The model under review builds one solid part; all positions refer to its coordinate system, in mm. Face numbers are marked on the shaded views. A direction names the side the tool comes from. Round coordinates to 2 decimals unless told otherwise and drop trailing zeros. Write each loop counter-clockwise with the first axis right and the second up, starting at its lowest first coordinate (ties: lowest second). Pieces come first, ordered by that corner, then holes. Notation, with made-up numbers: (24, 63.5) - (76, 63.5) arc R28 cw to (76, 96.5) - close; hole circle Ø4 at (38.5, 55.5). An arc over 180 degrees is marked (long way). Return JSON: item names as keys, results as strings.
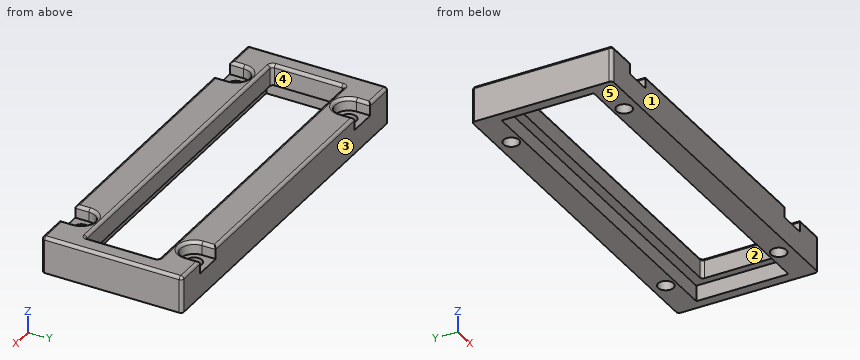
from build123d import *

# Parameters (mm, degrees)
SKETCH1_W                                      = 63.5
SKETCH1_H                                      = 24.384
BOSS_EXTRUDE1_DEPTH                            = 6.35
CBORE_FOR_2_SOCKET_HEAD_CAP_SCREW1_D           = 2.7051
CBORE_FOR_2_SOCKET_HEAD_CAP_SCREW1_CBORE_D     = 4.7625
CBORE_FOR_2_SOCKET_HEAD_CAP_SCREW1_CBORE_DEPTH = 2.1844
SKETCH4_W                                      = 57.404
SKETCH4_H                                      = 12.7
CUT_EXTRUDE1_DEPTH                             = 7.35
SKETCH5_W                                      = 4.7625
SKETCH5_H                                      = 2.3876
CUT_EXTRUDE2_DEPTH                             = 2.1844
SKETCH7_W                                      = 57.404
SKETCH7_H                                      = 12.7
CUT_EXTRUDE3_DEPTH                             = 2.7432
FILLET1_R                                      = 0.508
SKETCH11_W                                     = 60
SKETCH11_H                                     = 16
CUT_EXTRUDE6_DEPTH                             = 3.7432
BOSS_EXTRUDE2_REACH                            = 8.35


with BuildPart() as part:
    # Sketch1 → Boss-Extrude1 (new body)
    with BuildSketch(Plane.XY):
        with Locations((137.237805359, -177.626597764)):
            Rectangle(SKETCH1_W, SKETCH1_H)
    extrude(amount=BOSS_EXTRUDE1_DEPTH)

    # CBORE for #2 Socket Head Cap Screw1 (through all)
    with Locations(Plane.XY.offset(6.35)):
        with Locations((161.050305359, -187.430997764), (113.425305359, -187.430997764), (161.050305359, -167.822197764), (113.425305359, -167.822197764)):
            CounterBoreHole(CBORE_FOR_2_SOCKET_HEAD_CAP_SCREW1_D / 2, CBORE_FOR_2_SOCKET_HEAD_CAP_SCREW1_CBORE_D / 2, CBORE_FOR_2_SOCKET_HEAD_CAP_SCREW1_CBORE_DEPTH)

    # Sketch4 → Cut-Extrude1 (cut, through all)
    with BuildSketch(Plane.XY.offset(6.35)):
        with Locations((137.237805359, -177.626597764)):
            Rectangle(SKETCH4_W, SKETCH4_H)
    extrude(amount=-CUT_EXTRUDE1_DEPTH, mode=Mode.SUBTRACT)

    # Sketch5 → Cut-Extrude2 (cut)
    with BuildSketch(Plane.XY.offset(6.35)):
        with Locations((113.425305359, -166.628397764)):
            Rectangle(SKETCH5_W, SKETCH5_H)
        with Locations((161.050305359, -166.628397764)):
            Rectangle(SKETCH5_W, SKETCH5_H)
        with Locations((113.425305359, -188.624797764)):
            Rectangle(SKETCH5_W, SKETCH5_H)
        with Locations((161.050305359, -188.624797764)):
            Rectangle(SKETCH5_W, SKETCH5_H)
    extrude(amount=-CUT_EXTRUDE2_DEPTH, mode=Mode.SUBTRACT)

    # Sketch7 → Cut-Extrude3 (cut)
    with BuildSketch(Plane(origin=(0, 0, 0), x_dir=(-1, 0, 0), z_dir=(0, 0, -1))):
        with BuildLine():
            Line((-163.431555359, -167.822197764), (-163.431555359, -166.704597764))
            Line((-163.431555359, -166.704597764), (-167.717805359, -166.704597764))
            Line((-167.717805359, -166.704597764), (-167.717805359, -188.548597764))
            Line((-167.717805359, -188.548597764), (-163.431555359, -188.548597764))
            Line((-163.431555359, -188.548597764), (-163.431555359, -187.430997764))
            ThreePointArc((-163.431555359, -187.430997764), (-161.050305359, -185.049747764), (-158.669055359, -187.430997764))
            Line((-158.669055359, -187.430997764), (-158.669055359, -188.548597764))
            Line((-158.669055359, -188.548597764), (-115.806555359, -188.548597764))
            Line((-115.806555359, -188.548597764), (-115.806555359, -187.430997764))
            ThreePointArc((-115.806555359, -187.430997764), (-113.425305359, -185.049747764), (-111.044055359, -187.430997764))
            Line((-111.044055359, -187.430997764), (-111.044055359, -188.548597764))
            Line((-111.044055359, -188.548597764), (-106.757805359, -188.548597764))
            Line((-106.757805359, -188.548597764), (-106.757805359, -166.704597764))
            Line((-106.757805359, -166.704597764), (-111.044055359, -166.704597764))
            Line((-111.044055359, -166.704597764), (-111.044055359, -167.822197764))
            ThreePointArc((-111.044055359, -167.822197764), (-113.425305359, -170.203447764), (-115.806555359, -167.822197764))
            Line((-115.806555359, -167.822197764), (-115.806555359, -166.704597764))
            Line((-115.806555359, -166.704597764), (-158.669055359, -166.704597764))
            Line((-158.669055359, -166.704597764), (-158.669055359, -167.822197764))
            ThreePointArc((-158.669055359, -167.822197764), (-161.050305359, -170.203447764), (-163.431555359, -167.822197764))
        make_face()
        with Locations((-137.237805359, -177.626597764)):
            Rectangle(SKETCH7_W, SKETCH7_H, mode=Mode.SUBTRACT)
    extrude(amount=-CUT_EXTRUDE3_DEPTH, mode=Mode.SUBTRACT)

    # Fillet1
    fillet1_edges = [part.edges().sort_by_distance(p)[0] for p in [
        (105.487805359, -177.626597764, 6.35),
        (166.209680359, -189.818597764, 6.35),
        (158.669055359, -188.624797764, 6.35),
        (163.431555359, -188.624797764, 6.35),
        (108.265930359, -189.818597764, 6.35),
        (108.535805359, -171.276597764, 4.5466),
        (165.939805359, -171.276597764, 4.5466),
        (108.535805359, -183.976597764, 4.5466),
        (165.939805359, -183.976597764, 4.5466),
        (106.757805359, -166.704597764, 1.3716),
        (111.044055359, -166.704597764, 1.3716),
        (115.806555359, -166.704597764, 1.3716),
        (113.425305359, -185.049747764, 6.35),
        (161.050305359, -185.049747764, 6.35),
        (168.987805359, -177.626597764, 6.35),
        (165.939805359, -177.626597764, 6.35),
        (137.237805359, -171.276597764, 6.35),
        (108.535805359, -177.626597764, 6.35),
        (137.237805359, -183.976597764, 6.35),
        (113.425305359, -170.203447764, 6.35),
        (108.265930359, -165.434597764, 6.35),
        (115.806555359, -166.628397764, 6.35),
        (111.044055359, -166.628397764, 6.35),
        (166.209680359, -165.434597764, 6.35),
        (168.987805359, -189.818597764, 3.175),
        (105.487805359, -189.818597764, 3.175),
        (161.050305359, -170.203447764, 6.35),
        (105.487805359, -165.434597764, 3.175),
        (168.987805359, -165.434597764, 3.175),
        (137.237805359, -165.434597764, 6.35),
        (163.431555359, -166.628397764, 6.35),
        (158.669055359, -166.628397764, 6.35),
        (137.237805359, -189.818597764, 6.35),
        (115.806555359, -188.624797764, 6.35),
        (111.044055359, -188.624797764, 6.35),
    ]]
    fillet(fillet1_edges, radius=FILLET1_R)

    # Sketch11 → Cut-Extrude6 (cut, through all)
    with BuildSketch(Plane(origin=(0, 0, 2.7432), x_dir=(-1, 0, 0), z_dir=(0, 0, -1))):
        with Locations((-137.237805359, -177.626597764)):
            Rectangle(SKETCH11_W, SKETCH11_H)
    extrude(amount=CUT_EXTRUDE6_DEPTH, mode=Mode.SUBTRACT)

    # Sketch10 → Boss-Extrude2 (add, up to next)
    with BuildSketch(Plane(origin=(0, 0, 0), x_dir=(-1, 0, 0), z_dir=(0, 0, -1)), mode=Mode.PRIVATE) as boss_extrude2_sk1:
        with BuildLine():
            ThreePointArc((-158.669055359, -167.822197764), (-158.885762757, -168.814723274), (-159.496441722, -169.626597764))
            Line((-159.496441722, -169.626597764), (-114.979168996, -169.626597764))
            ThreePointArc((-114.979168996, -169.626597764), (-115.58984796, -168.814723274), (-115.806555359, -167.822197764))
            Line((-115.806555359, -167.822197764), (-115.806555359, -167.212597764))
            ThreePointArc((-115.806555359, -167.212597764), (-115.955345114, -166.853387519), (-116.314555359, -166.704597764))
            Line((-116.314555359, -166.704597764), (-158.669055359, -166.704597764))
            Line((-158.669055359, -166.704597764), (-158.669055359, -167.822197764))
        make_face()
    boss_extrude2_tool1 = extrude(boss_extrude2_sk1.sketch, amount=-BOSS_EXTRUDE2_REACH, mode=Mode.PRIVATE) - part.part
    add(boss_extrude2_tool1.solids().sort_by_distance((137.247168, -168.173633, 0))[0])
    # Sketch10 → Boss-Extrude2 (add, up to next)
    with BuildSketch(Plane(origin=(0, 0, 0), x_dir=(-1, 0, 0), z_dir=(0, 0, -1)), mode=Mode.PRIVATE) as boss_extrude2_sk2:
        with BuildLine():
            Line((-107.237805359, -185.626597764), (-111.871441722, -185.626597764))
            ThreePointArc((-111.871441722, -185.626597764), (-111.260762757, -186.438472254), (-111.044055359, -187.430997764))
            Line((-111.044055359, -187.430997764), (-111.044055359, -188.548597764))
            Line((-111.044055359, -188.548597764), (-106.757805359, -188.548597764))
            Line((-106.757805359, -188.548597764), (-106.757805359, -167.212597764))
            ThreePointArc((-106.757805359, -167.212597764), (-106.906595114, -166.853387519), (-107.265805359, -166.704597764))
            Line((-107.265805359, -166.704597764), (-110.536055359, -166.704597764))
            ThreePointArc((-110.536055359, -166.704597764), (-110.895265604, -166.853387519), (-111.044055359, -167.212597764))
            Line((-111.044055359, -167.212597764), (-111.044055359, -167.822197764))
            ThreePointArc((-111.044055359, -167.822197764), (-111.260762757, -168.814723274), (-111.871441722, -169.626597764))
            Line((-111.871441722, -169.626597764), (-107.237805359, -169.626597764))
            Line((-107.237805359, -169.626597764), (-107.237805359, -185.626597764))
        make_face()
    boss_extrude2_tool2 = extrude(boss_extrude2_sk2.sketch, amount=-BOSS_EXTRUDE2_REACH, mode=Mode.PRIVATE) - part.part
    add(boss_extrude2_tool2.solids().sort_by_distance((111.056834, -186.344963, 0))[0])
    # Sketch10 → Boss-Extrude2 (add, up to next)
    with BuildSketch(Plane(origin=(0, 0, 0), x_dir=(-1, 0, 0), z_dir=(0, 0, -1)), mode=Mode.PRIVATE) as boss_extrude2_sk3:
        with BuildLine():
            Line((-114.979168996, -185.626597764), (-159.496441722, -185.626597764))
            ThreePointArc((-159.496441722, -185.626597764), (-158.885762757, -186.438472254), (-158.669055359, -187.430997764))
            Line((-158.669055359, -187.430997764), (-158.669055359, -188.548597764))
            Line((-158.669055359, -188.548597764), (-115.806555359, -188.548597764))
            Line((-115.806555359, -188.548597764), (-115.806555359, -187.430997764))
            ThreePointArc((-115.806555359, -187.430997764), (-115.58984796, -186.438472254), (-114.979168996, -185.626597764))
        make_face()
    boss_extrude2_tool3 = extrude(boss_extrude2_sk3.sketch, amount=-BOSS_EXTRUDE2_REACH, mode=Mode.PRIVATE) - part.part
    add(boss_extrude2_tool3.solids().sort_by_distance((137.237805, -187.080157, 0))[0])
    # Sketch10 → Boss-Extrude2 (add, up to next)
    with BuildSketch(Plane(origin=(0, 0, 0), x_dir=(-1, 0, 0), z_dir=(0, 0, -1)), mode=Mode.PRIVATE) as boss_extrude2_sk4:
        with BuildLine():
            Line((-162.604168996, -185.626597764), (-167.237805359, -185.626597764))
            Line((-167.237805359, -185.626597764), (-167.237805359, -169.626597764))
            Line((-167.237805359, -169.626597764), (-162.604168996, -169.626597764))
            ThreePointArc((-162.604168996, -169.626597764), (-163.21484796, -168.814723274), (-163.431555359, -167.822197764))
            Line((-163.431555359, -167.822197764), (-163.431555359, -166.704597764))
            Line((-163.431555359, -166.704597764), (-167.717805359, -166.704597764))
            Line((-167.717805359, -166.704597764), (-167.717805359, -188.548597764))
            Line((-167.717805359, -188.548597764), (-163.431555359, -188.548597764))
            Line((-163.431555359, -188.548597764), (-163.431555359, -187.430997764))
            ThreePointArc((-163.431555359, -187.430997764), (-163.21484796, -186.438472254), (-162.604168996, -185.626597764))
        make_face()
    boss_extrude2_tool4 = extrude(boss_extrude2_sk4.sketch, amount=-BOSS_EXTRUDE2_REACH, mode=Mode.PRIVATE) - part.part
    add(boss_extrude2_tool4.solids().sort_by_distance((164.920987, -185.850943, 0))[0])


solid = part.part
(1) Add section B-B (x = 118). Write out the cut boundary in (y, z), plus the area to 3 significant figures.
Filled in:
{"outline": "(-189.82, 0) - (-185.63, 0) - (-185.63, 2.74) - (-183.98, 2.74) - (-183.98, 5.84) arc R0.51 ccw to (-184.48, 6.35) - (-189.31, 6.35) arc R0.51 ccw to (-189.82, 5.84) - close; (-171.28, 2.74) - (-169.63, 2.74) - (-169.63, 0) - (-165.43, 0) - (-165.43, 5.84) arc R0.51 ccw to (-165.94, 6.35) - (-170.77, 6.35) arc R0.51 ccw to (-171.28, 5.84) - close", "area": "64.9 mm2"}
(2) Wall thickness on line 1 (Y direction, x = 163, z = 4); line 2 (X direction, y = -182.5, z = 2); line 3 (Y direction, x = 120.5, z = 1.5): over which ranges is each line inside the solid? List them lowest first.
Filled in:
{"line 1": "y = -189.82 to -183.98, -171.28 to -165.43", "line 2": "x = 105.49 to 107.24, 167.24 to 168.99", "line 3": "y = -189.82 to -185.63, -169.63 to -165.43"}
(3) Mouldability with a two-part tool opening along Y and no side actions: class the marked faces 3, 4 and 5 as released by +Y, released by -Y, zero draft, split by the parting line, or undercut.
Filled in:
{"face 3": "released by +Y", "face 4": "undercut", "face 5": "zero draft"}
(4) Add section C-C (z = 1.25). Write out the cut boundary in (x, y).
Filled in:
{"outline": "(105.49, -189.31) arc R0.51 ccw to (106, -189.82) - (168.48, -189.82) arc R0.51 ccw to (168.99, -189.31) - (168.99, -165.94) arc R0.51 ccw to (168.48, -165.43) - (106, -165.43) arc R0.51 ccw to (105.49, -165.94) - close; hole (107.24, -185.63) - (167.24, -185.63) - (167.24, -169.63) - (107.24, -169.63) - close; hole circle Ø2.71 at (113.43, -187.43); hole circle Ø2.71 at (113.43, -167.82); hole circle Ø2.71 at (161.05, -187.43); hole circle Ø2.71 at (161.05, -167.82)"}
(5) For the marked faces 1 and 2, list the 3-axis set-ups (+Z, -Z, +X, -X, +Y, -Y) from which the entire face can be reached by the end or side of a thin tool; tool diameter is ignored.
Filled in:
{"face 1": "+Z, -Z, +X, -X, -Y", "face 2": "+Z, -Z"}
(6) Clearance check with flat-ended pins moving along their axes: pin 1 Ø8 at (x, y) = (137.5, -177.5) entering from -Z; pin 2 Ø10 at (x, y) = (114, -168.5) entering from -Z; pin 3 Ø1.4 at (x, y) = (160, -168) entering from +Z. State where each tip first meets the part, or that it passes through.
Filled in:
{"pin 1": "passes through", "pin 2": "stops at z = 0", "pin 3": "stops at z = 4.17"}
(7) Add section A-A (y = -181.5). Write out the cut boundary in (x, z), plus the area to 3 significant figures.
Filled in:
{"outline": "(105.49, 0) - (107.24, 0) - (107.24, 2.74) - (108.54, 2.74) - (108.54, 5.84) arc R0.51 ccw to (108.03, 6.35) - (106, 6.35) arc R0.51 ccw to (105.49, 5.84) - close; (165.94, 2.74) - (167.24, 2.74) - (167.24, 0) - (168.99, 0) - (168.99, 5.84) arc R0.51 ccw to (168.48, 6.35) - (166.45, 6.35) arc R0.51 ccw to (165.94, 5.84) - close", "area": "31.4 mm2"}
